The listing builds one solid part. Answer for the finished solid, in the listing's coordinates (mm). A direction names the side the tool comes from. Round coordinates to 2 decimals unless told otherwise and drop trailing zeros. Loops run counter-clockwise (first coordinate to the right, second up) from the corner with the lowest first, then second, coordinate; pieces in that order, holes last. Notation, with made-up numbers: (85.25, -6) -> (120.25, -6) arc R21 ccw to (120.25, 22) -> close; hole circle Ø2 at (-7.5, 85). An arc over 180 degrees is marked (long way). One line per question, with ' | ' between items.
from build123d import *

# Parameters (mm, degrees)
BOSS_EXTRUDE1_DEPTH = 14.54
BOSS_EXTRUDE2_DEPTH = 1.6
SKETCH5_W           = 12.35
SKETCH5_H           = 4.1
BOSS_EXTRUDE3_DEPTH = 2.45


with BuildPart() as part:
    # Sketch1 → Boss-Extrude1 (new body)
    with BuildSketch(Plane(origin=(0, 0, 0), x_dir=(1, 0, 0), z_dir=(0, 1, 0))):
        with BuildLine():
            Line((-6.529165337, -5.72), (6.529165337, -5.72))
            ThreePointArc((6.529165337, -5.72), (7.849312473, -5.343019439), (8.771323763, -4.325769231))
            ThreePointArc((8.771323763, -4.325769231), (0, 9.78), (-8.771323763, -4.325769231))
            ThreePointArc((-8.771323763, -4.325769231), (-7.849312473, -5.343019439), (-6.529165337, -5.72))
        make_face()
    extrude(amount=BOSS_EXTRUDE1_DEPTH)

    # Sketch3 → Boss-Extrude2 (add)
    with BuildSketch(Plane.XZ):
        with BuildLine():
            Line((6.529165337, 6.35), (-6.529165337, 6.35))
            ThreePointArc((-6.529165337, 6.35), (-8.181989552, 5.878020338), (-9.336347687, 4.604423077))
            ThreePointArc((-9.336347687, 4.604423077), (0, -10.41), (9.336347687, 4.604423077))
            ThreePointArc((9.336347687, 4.604423077), (8.181989552, 5.878020338), (6.529165337, 6.35))
        make_face()
    extrude(amount=BOSS_EXTRUDE2_DEPTH)

    # Sketch5 → Boss-Extrude3 (add)
    with BuildSketch(Plane.XZ.offset(1.6)):
        Rectangle(SKETCH5_W, SKETCH5_H)
    extrude(amount=BOSS_EXTRUDE3_DEPTH)


solid = part.part
Q1. A cutting plane is placed at B-B on z = 0. Give the vertices of the cut face in (x, y) (3 decimals), plus the area to 3 significant figures.
Numbers:
outline: (-10.41, -1.6) -> (-6.175, -1.6) -> (-6.175, -4.05) -> (6.175, -4.05) -> (6.175, -1.6) -> (10.41, -1.6) -> (10.41, 0) -> (9.78, 0) -> (9.78, 14.54) -> (-9.78, 14.54) -> (-9.78, 0) -> (-10.41, 0) -> close | area: 348 mm^2
Q2. A cutting plane is placed at D-D on z = -8. Give the vertices of the cut face in (x, y).
Numbers:
outline: (-6.66, -1.6) -> (6.66, -1.6) -> (6.66, 0) -> (5.63, 0) -> (5.63, 14.54) -> (-5.63, 14.54) -> (-5.63, 0) -> (-6.66, 0) -> close
Q3. For faces 1 (the face through (7.833, 7.168, 5.353)), 2 (the face through (6.175, -3, 0)), 3 (the face through (0, -3, -2.05)), 4 (the face through (-7.87, 7.17, 5.33)), determine the directions among +Z, -Z, +X, -X, +Y, -Y from which every point of the face is accessible in a straight line to the end or side of a thin tool.
Numbers:
face 1: +Z, +X, +Y | face 2: +Z, -Z, +X, -Y | face 3: -Z, +X, -X, -Y | face 4: +Z, -X, +Y
Q4. Find the intervals of material crossed by line 1 (X direction, y = 9.25, z = -0.25); line 2 (Y direction, x = -2.5, z = 5.75); line 3 (Y direction, x = -4.25, z = -4), in increasing order. Write a range as from..to.
Numbers:
line 1: -9.78..9.78 | line 2: -1.6..0 | line 3: -1.6..14.54
Q5. A cutting plane is placed at A-A on x = 0. Give the vertices of the cut face in (y, z).
Numbers:
outline: (-4.05, -2.05) -> (-1.6, -2.05) -> (-1.6, -10.41) -> (0, -10.41) -> (0, -9.78) -> (14.54, -9.78) -> (14.54, 5.72) -> (0, 5.72) -> (0, 6.35) -> (-1.6, 6.35) -> (-1.6, 2.05) -> (-4.05, 2.05) -> close
Q6. A cutting plane is placed at C-C on y = -2.5. Give the vertices of the cut face in (x, z) (3 decimals).
Numbers:
outline: (-6.175, -2.05) -> (6.175, -2.05) -> (6.175, 2.05) -> (-6.175, 2.05) -> close
Q7. Given pin 1 Ø3 at (y, z) = (12, -7.5) entering from -X; pin 2 Ø2.5 at (x, y) = (1.5, -3) entering from +Z; pin 3 Ø8 at (y, z) = (3.5, 3.5) entering from -X, each flat-ended and moving along its own axis, determine where each tip first touches the part or whether it passes through.
Numbers:
pin 1: x = -7.72 | pin 2: z = 2.05 | pin 3: x = -10.29
